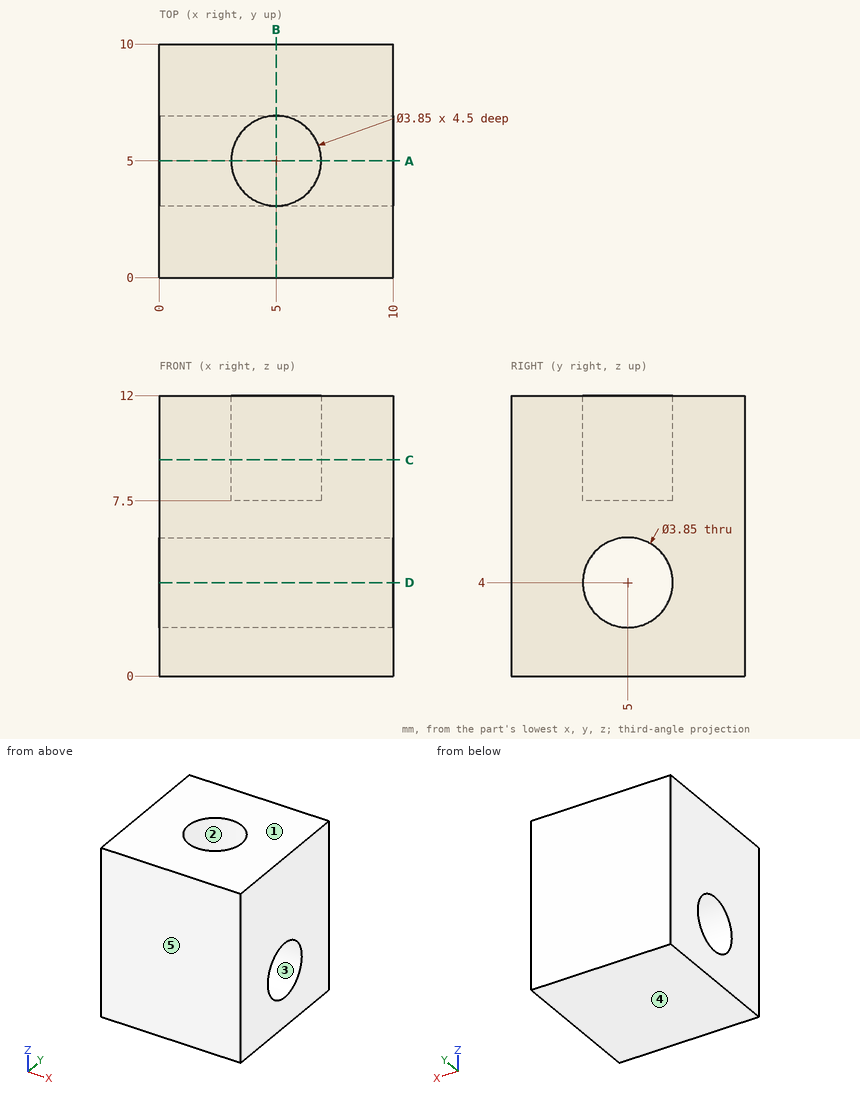
The figure shows three views and two pictorial views of one solid part (mm, origin at its lowest corner). Answer the questions. A direction names the side the tool comes from. Give positions to 0.01 mm unless a question says otherwise; leave off trailing zeros. Write each loop counter-clockwise with the first axis right and the second up, starting at its lowest first coordinate (ties: lowest second). Pieces come first, ordered by that corner, then holes.
Q1. For a pull along Y with two mould halves and no side action, classify the marked faces 3, 4 and 5 as released by +Y, released by -Y, zero draft, split by the parting line, or undercut.
Answer:
face 3: undercut
face 4: zero draft
face 5: released by -Y
Q2. The part is cut by section B-B on x = 5. Give the vertices of the cut face in (y, z) (3 decimals), and give its area (3 significant figures).
Answer:
outline: (0, 0) - (10, 0) - (10, 12) - (6.925, 12) - (6.925, 7.5) - (3.075, 7.5) - (3.075, 12) - (0, 12) - close; hole circle Ø3.85 at (5, 4)
area: 91.0 mm2
Q3. The part is cut by section A-A on y = 5. Give the vertices of the cut face in (x, z) (3 decimals).
Answer:
outline: (0, 0) - (10, 0) - (10, 2.075) - (0, 2.075) - close; (0, 5.925) - (10, 5.925) - (10, 12) - (6.925, 12) - (6.925, 7.5) - (3.075, 7.5) - (3.075, 12) - (0, 12) - close
Q4. Straight lines are drawn through the part: L1, parallel to Y at x = 6.5, z = 4 (3 decimals); L2, parallel to Y at x = 3.5, z = 8.25; L3, parallel to Z at x = 2.25, y = 6.5. For each, find the intervals that lie inside material, in ascending order.
Answer:
L1: y = 0 to 3.075, 6.925 to 10
L2: y = 0 to 3.79, 6.21 to 10
L3: z = 0 to 2.79, 5.21 to 12
Q5. The part is cut by section C-C on z = 9.25. Give the vertices of the cut face in (x, y) (3 decimals).
Answer:
outline: (0, 0) - (10, 0) - (10, 10) - (0, 10) - close; hole circle Ø3.85 at (5, 5)
Q6. A tool of negligible diameter and unlimited length cuts with its end or side. For the marked faces 1 and 2, from which of +Z, -Z, +X, -X, +Y, -Y can it reach the whole face along a straight path? Write none if from no direction.
Answer:
face 1: +Z, +X, -X, +Y, -Y
face 2: +Z
Q7. The part is cut by section D-D on z = 4. Give the vertices of the cut face in (x, y) (3 decimals), and give its area (3 significant figures).
Answer:
outline: (0, 0) - (10, 0) - (10, 3.075) - (0, 3.075) - close; (0, 6.925) - (10, 6.925) - (10, 10) - (0, 10) - close
area: 61.5 mm2
Q8. Given pin 1 (1.9 mm diameter, centred on x = 5.5, y = 4.5, fed in from +Z), flat-ended and moving along its own axis, determine where the tip first touches the part or whether it passes through.
Answer:
pin 1: stops at z = 7.5
